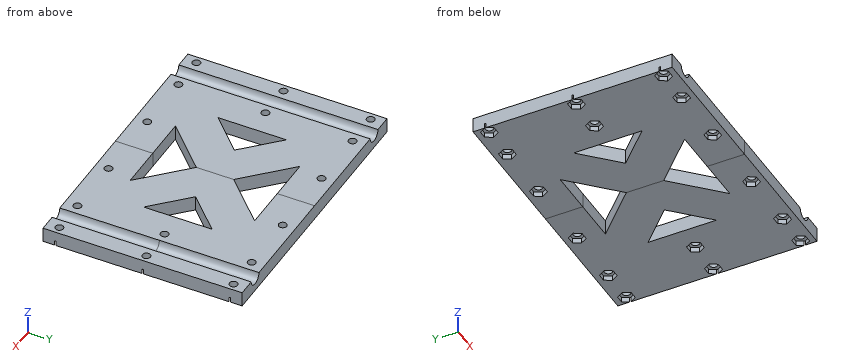
from build123d import *

# Parameters (mm, degrees)
SKETCH_R          = 1.6
PAD_DEPTH         = 6
SKETCH001_R       = 3
POCKET_DEPTH      = 40.001
POCKET_DEPTH_BACK = -40.001
POCKET001_DEPTH   = 2


with BuildPart() as toolbody:
    # Sketch → Pad (new body)
    with BuildSketch(Plane.XY):
        Polygon((0, 40), (46, 40), (56, 40), (56, -40), (46, -40), (0, -40), (0, -25), (17.5, -25), (0, -7.5), (0, 7.5), (17.5, 25), (0, 25), align=None)
        with Locations((53, 0)):
            Circle(SKETCH_R, mode=Mode.SUBTRACT)
        with Locations((53, 35)):
            Circle(SKETCH_R, mode=Mode.SUBTRACT)
        with Locations((53, -35)):
            Circle(SKETCH_R, mode=Mode.SUBTRACT)
        with Locations((39, 35)):
            Circle(SKETCH_R, mode=Mode.SUBTRACT)
        with Locations((39, 0)):
            Circle(SKETCH_R, mode=Mode.SUBTRACT)
        with Locations((39, -35)):
            Circle(SKETCH_R, mode=Mode.SUBTRACT)
        with Locations((15, 35)):
            Circle(SKETCH_R, mode=Mode.SUBTRACT)
        with Locations((15, -35)):
            Circle(SKETCH_R, mode=Mode.SUBTRACT)
        Polygon((15, 0), (28.75, 13.75), (28.75, -13.75), align=None, mode=Mode.SUBTRACT)
    extrude(amount=-PAD_DEPTH)

    # Sketch001 → Pocket (cut, two sides)
    with BuildSketch(Plane.XZ) as pocket_sk:
        with Locations((46, 0)):
            Circle(SKETCH001_R)
    extrude(amount=-POCKET_DEPTH, mode=Mode.SUBTRACT)
    extrude(pocket_sk.sketch, amount=-POCKET_DEPTH_BACK, mode=Mode.SUBTRACT)

    # Sketch002 (on DatumPlane) → Pocket001 (cut)
    with BuildSketch(Plane.XY.offset(-6)):
        Polygon((16.587713, 32.25), (18.175426, 35), (16.587713, 37.75), (13.412287, 37.75), (11.824574, 35), (13.412287, 32.25), align=None)
        Polygon((40.587713, 32.25), (42.175426, 35), (40.587713, 37.75), (37.412287, 37.75), (35.824574, 35), (37.412287, 32.25), align=None)
        Polygon((54.587713, 32.25), (56.175426, 35), (54.587713, 37.75), (51.412287, 37.75), (49.824574, 35), (51.412287, 32.25), align=None)
        Polygon((54.587713, -2.75), (56.175426, 0), (54.587713, 2.75), (51.412287, 2.75), (49.824574, 0), (51.412287, -2.75), align=None)
        Polygon((40.587713, -2.75), (42.175426, 0), (40.587713, 2.75), (37.412287, 2.75), (35.824574, 0), (37.412287, -2.75), align=None)
        Polygon((54.587713, -37.75), (56.175426, -35), (54.587713, -32.25), (51.412287, -32.25), (49.824574, -35), (51.412287, -37.75), align=None)
        Polygon((40.587713, -37.75), (42.175426, -35), (40.587713, -32.25), (37.412287, -32.25), (35.824574, -35), (37.412287, -37.75), align=None)
        Polygon((16.587713, -37.75), (18.175426, -35), (16.587713, -32.25), (13.412287, -32.25), (11.824574, -35), (13.412287, -37.75), align=None)
    extrude(amount=POCKET001_DEPTH, mode=Mode.SUBTRACT)


with BuildPart() as toolfusion:
    # Part__Mirroring: instance of ToolBody
    add(toolbody.part.mirror(Plane(origin=(0, 0, 0), x_dir=(0, -1, 0), z_dir=(1, 0, 0))))

    # Fusion: union ToolBody
    add(toolbody.part)


solid = toolfusion.part
Check sheet for the modelled part. Datum: model origin and axes. Units: mm. Give positions to 0.01 mm unless a question says otherwise; leave off trailing zeros. Write each loop counter-clockwise with the first axis right and the second up, starting at its lowest first coordinate (ties: lowest second). Pieces come first, ordered by that corner, then holes. Notation, with made-up numbers: (40.25, 85.25) -> (59.25, 85.25) arc R32 ccw to (59.25, 120.25) -> close; hole circle Ø1 at (62, 57). An arc over 180 degrees is marked (long way). Write item = value, one per line.
Item 1: Sectioned sample at A-A on x = 53. Record the boundary of the cut face in (y, z).
Output:
outline = (-40, -6) -> (-37.75, -6) -> (-37.75, -4) -> (-36.6, -4) -> (-36.6, 0) -> (-40, 0) -> close; (-33.4, -4) -> (-32.25, -4) -> (-32.25, -6) -> (-2.75, -6) -> (-2.75, -4) -> (-1.6, -4) -> (-1.6, 0) -> (-33.4, 0) -> close; (1.6, -4) -> (2.75, -4) -> (2.75, -6) -> (32.25, -6) -> (32.25, -4) -> (33.4, -4) -> (33.4, 0) -> (1.6, 0) -> close; (36.6, -4) -> (37.75, -4) -> (37.75, -6) -> (40, -6) -> (40, 0) -> (36.6, 0) -> close
Item 2: Gauge pin test, flat ends, axial feed: pin 1 (6 mm diameter, centred on x = -40, y = -34.5, fed in from -Z); pin 2 (4 mm diameter, centred on x = -53, y = 35, fed in from -Z). Record the tip position at first contact, or that the pin passes through.
Output:
pin_1 = -6
pin_2 = -4
Item 3: Scan lines: probe 1 along Y at (x, z) = (-53, -2.1); probe 2 along Y at (x, z) = (5.5, -3.55); probe 3 along Y at (x, z) = (4.5, -4.75). Record each from-to range of solid material in increasing order. Write a range as from..to.
Output:
probe_1 = -40..-36.6, -33.4..-1.6, 1.6..33.4, 36.6..40
probe_2 = -40..-25, -13..13, 25..40
probe_3 = -40..-25, -12..12, 25..40
Item 4: Sectioned sample at D-D on x = 26. Record the boundary of the cut face in (y, z).
Output:
outline = (-40, -6) -> (-11, -6) -> (-11, 0) -> (-40, 0) -> close; (11, -6) -> (40, -6) -> (40, 0) -> (11, 0) -> close
Item 5: Sectioned sample at B-B on y = 19. Record the boundary of the cut face in (x, z).
Output:
outline = (-56, -6) -> (-11.5, -6) -> (-11.5, 0) -> (-43, 0) arc R3 cw to (-49, 0) -> (-56, 0) -> close; (11.5, -6) -> (56, -6) -> (56, 0) -> (49, 0) arc R3 cw to (43, 0) -> (11.5, 0) -> close
Item 6: Sectioned sample at C-C on x = -2.5. Record the boundary of the cut face in (y, z).
Output:
outline = (-40, -6) -> (-25, -6) -> (-25, 0) -> (-40, 0) -> close; (-10, -6) -> (10, -6) -> (10, 0) -> (-10, 0) -> close; (25, -6) -> (40, -6) -> (40, 0) -> (25, 0) -> close
